```python
from build123d import *

# Parameters (mm, degrees)
BOSS_EXTRUDE1_DEPTH = 16.25
CUT_EXTRUDE1_DEPTH  = 1
SKETCH3_R           = 3.825
BOSS_EXTRUDE2_DEPTH = 3
CUT_EXTRUDE2_DEPTH  = 25.3
FILLET1_R           = 0.2
FILLET2_R           = 0.5
FILLET3_R           = 3
CUT_EXTRUDE3_DEPTH  = 4.45
CHAMFER1_SIZE       = 1.5


with BuildPart() as part:
    # Sketch1 → Boss-Extrude1 (new body, symmetric)
    with BuildSketch(Plane(origin=(0, 0, 0), x_dir=(0, 0, -1), z_dir=(1, 0, 0))):
        with BuildLine():
            Line((0, 0), (37.222256431, 0))
            ThreePointArc((37.222256431, 0), (44.515232504, 2.608290378), (48.5, 9.25))
            Line((48.5, 9.25), (44.35, 9.8))
            Line((44.35, 9.8), (44.35, 13.2))
            Line((44.35, 13.2), (48.5, 13.75))
            ThreePointArc((48.5, 13.75), (45.353984415, 19.631727984), (39.472256431, 22.777743569))
            Line((39.472256431, 22.777743569), (38.922256431, 18.627743569))
            Line((38.922256431, 18.627743569), (35.522256431, 18.627743569))
            Line((35.522256431, 18.627743569), (34.972256431, 22.777743569))
            ThreePointArc((34.972256431, 22.777743569), (30.886246606, 21.097133921), (27.735423451, 18))
            Line((27.735423451, 18), (0, 11.626817203))
            Line((0, 11.626817203), (0, 0))
        make_face()
    extrude(amount=BOSS_EXTRUDE1_DEPTH, both=True)

    # Sketch2 → Cut-Extrude1 (cut)
    with BuildSketch(Plane(origin=(16.25, 0, 0), x_dir=(0, 0, -1), z_dir=(1, 0, 0))):
        Polygon((24.85, 17.336973126), (24.85, 0), (48.5, 0), (48.5, 22.777743569), (24.85, 22.777743569), align=None)
    cut_extrude1 = extrude(amount=-CUT_EXTRUDE1_DEPTH, mode=Mode.SUBTRACT)

    # Sketch3 → Boss-Extrude2 (add)
    with BuildSketch(Plane(origin=(15.25, 0, 0), x_dir=(0, 0, -1), z_dir=(1, 0, 0))):
        with Locations((37.222256431, 11.5)):
            Circle(SKETCH3_R)
    boss_extrude2 = extrude(amount=BOSS_EXTRUDE2_DEPTH)

    # Mirror1: Cut-Extrude1, Boss-Extrude2 across plane
    add(cut_extrude1.mirror(Plane(origin=(0, 0, 0), x_dir=(0, 0, 1), z_dir=(1, 0, 0))), mode=Mode.SUBTRACT)
    add(boss_extrude2.mirror(Plane(origin=(0, 0, 0), x_dir=(0, 0, 1), z_dir=(1, 0, 0))))

    # Sketch4 → Cut-Extrude2 (cut)
    with BuildSketch(Plane(origin=(12.65, 0, 0), x_dir=(0, 0, -1), z_dir=(1, 0, 0))):
        Polygon((0, 1.1), (1.35, 1.1), (1.35, 2.7), (2.65, 2.7), (2.65, 0), (0, 0), align=None)
        Polygon((0, 3.45), (27, 3.45), (31.5, 0), (48.5, 0), (48.5, 22.777743569), (0, 22.777743569), align=None)
    extrude(amount=-CUT_EXTRUDE2_DEPTH, mode=Mode.SUBTRACT)

    # Fillet1
    fillet1_edges = [part.edges().sort_by_distance(p)[0] for p in [
        (-18.25, 11.5, -33.397256431),
        (18.25, 11.5, -33.397256431),
    ]]
    fillet(fillet1_edges, radius=FILLET1_R)

    # Fillet2
    fillet2_edges = [part.edges().sort_by_distance(p)[0] for p in [
        (-14.45, 0, 0),
        (-13.95, 22.777743569, -34.972256431),
        (-13.95, 22.777743569, -39.472256431),
        (-13.95, 13.75, -48.5),
        (-13.95, 9.25, -48.5),
        (14.45, 0, 0),
        (13.95, 22.777743569, -34.972256431),
        (13.95, 22.777743569, -39.472256431),
        (13.95, 13.75, -48.5),
        (13.95, 9.25, -48.5),
    ]]
    fillet(fillet2_edges, radius=FILLET2_R)

    # Fillet3
    fillet3_edges = [part.edges().sort_by_distance(p)[0] for p in [
        (-14.45, 11.626817203, 0),
        (14.45, 11.626817203, 0),
    ]]
    fillet(fillet3_edges, radius=FILLET3_R)

    # Sketch5 → Cut-Extrude3 (cut, through all)
    with BuildSketch(Plane(origin=(0, 3.45, 0), x_dir=(1, 0, 0), z_dir=(0, 1, 0))):
        with BuildLine():
            Line((-0.75, 4.75), (0.75, 4.75))
            ThreePointArc((0.75, 4.75), (3.5, 7.5), (0.75, 10.25))
            Line((0.75, 10.25), (-0.75, 10.25))
            ThreePointArc((-0.75, 10.25), (-3.5, 7.5), (-0.75, 4.75))
        make_face()
        with BuildLine():
            Line((7.75, 20.5), (6.25, 20.5))
            ThreePointArc((6.25, 20.5), (3.5, 17.75), (6.25, 15))
            Line((6.25, 15), (7.75, 15))
            ThreePointArc((7.75, 15), (10.5, 17.75), (7.75, 20.5))
        make_face()
        with BuildLine():
            Line((-7.75, 20.5), (-6.25, 20.5))
            ThreePointArc((-6.25, 20.5), (-3.5, 17.75), (-6.25, 15))
            Line((-6.25, 15), (-7.75, 15))
            ThreePointArc((-7.75, 15), (-10.5, 17.75), (-7.75, 20.5))
        make_face()
    extrude(amount=-CUT_EXTRUDE3_DEPTH, mode=Mode.SUBTRACT)

    # Chamfer1
    chamfer1_edges = [part.edges().sort_by_distance(p)[0] for p in [
        (-3.5, 3.45, -7.5),
        (0, 3.45, -4.75),
        (3.5, 3.45, -7.5),
        (0, 3.45, -10.25),
        (10.5, 3.45, -17.75),
        (7, 3.45, -20.5),
        (3.5, 3.45, -17.75),
        (7, 3.45, -15),
        (-10.5, 3.45, -17.75),
        (-7, 3.45, -15),
        (-3.5, 3.45, -17.75),
        (-7, 3.45, -20.5),
    ]]
    chamfer(chamfer1_edges, length=CHAMFER1_SIZE)


solid = part.part
```
Model file for the job. Use its own axes, mm. A direction names the side the tool comes from. Give positions to 0.01 mm unless a question says otherwise; leave off trailing zeros. Order: outer loops, then holes, each group sorted by start corner. A loop starts at its lowest first (then second) coordinate and runs counter-clockwise, first axis right, second up.
1) Saw through at A-A, the plane y = 6.5. Write the cut outline in (x, z).
2) Saw through at C-C, the plane z = -30.5. Write the cut outline in (x, y), then the cut area to 3 significant figures.
3) Saw through at B-B, the plane z = -7.5. Write the cut outline in (x, y).
4) Wall check: probe 1 along X at (y, z) = (16.75, -32.5); probe 2 along X at (y, z) = (10.75, -17); probe 3 along Z at (x, y) = (-8.5, 2.25). Give the ranges that are in metal, low to high.
5) Mould opens along Y. For faces 4 (the flat face through (-14, 11, -44.35)), 5 (the flat face through (16, 9, -24.85)), 6 (the cylindrical face through (-13.932, 2.368, -44.213)), 7 (the flat face through (-6.99, 2.69, -14.26)) say: +Y half, -Y half, draft (parallel to the pull), parting line (faces both ways), or undercut.
6) Saw through at D-D, the plane y = 11.5. Write the cut outline in (x, z), then the cut area to 3 significant figures.
7) 3-axis set-ups, long thin cutter, end or side, ignore diameter. For faces 1 (the conical face through (3.74, 2.19, -7.43)), 2 (the flat face through (0, 1, -10.25)), 3 (the flat face through (0, 2, -1.35)): which of +Z, -Z, +X, -X, +Y, -Y reach the whole face in a straight line?
8) Pin check, flat tips, straight feed: pin 1 (1.2 mm diameter, centred on x = 7, y = 1, fed in from -Z); pin 2 (6 mm diameter, centred on y = 11, z = -23.5, fed in from +X); pin 3 (2 mm diameter, centred on x = 0.5, z = -33, fed in from -Y); pin 4 (5 mm diameter, centred on y = 5.5, z = -13.5, fed in from -X). Stop position of each tip, or through.
Computed:
1. outline: (-16.25, -24.85) - (-15.25, -24.85) - (-15.25, -47.58) - (-12.65, -47.58) - (-12.65, 0) - (-16.25, 0) - close; (12.65, -47.58) - (15.25, -47.58) - (15.25, -24.85) - (16.25, -24.85) - (16.25, 0) - (12.65, 0) - close
2. outline: (-15.25, 0) - (15.25, 0) - (15.25, 20.83) - (12.65, 20.83) - (12.65, 0.77) - (-12.65, 0.77) - (-12.65, 20.83) - (-15.25, 20.83) - close
2. area: 128 mm2
3. outline: (-16.25, 0) - (-3.5, 0) - (-3.5, 1.95) - (-5, 3.45) - (-12.65, 3.45) - (-12.65, 13.35) - (-16.25, 13.35) - close; (3.5, 0) - (16.25, 0) - (16.25, 13.35) - (12.65, 13.35) - (12.65, 3.45) - (5, 3.45) - (3.5, 1.95) - close
4. probe 1: x = -15.25 to -12.65, 12.65 to 15.25
4. probe 2: x = -16.25 to -12.65, 12.65 to 16.25
4. probe 3: z = -28.57 to -20.71, -14.79 to -2.65, -1.35 to 0
5. face 4: undercut
5. face 5: draft
5. face 6: -Y half
5. face 7: +Y half
6. outline: (-18.25, -40.85) arc R0.2 ccw to (-18.05, -41.05) - (-15.25, -41.05) - (-15.25, -44.35) - (-12.65, -44.35) - (-12.65, -1.03) - (-16.25, -1.03) - (-16.25, -24.85) - (-15.25, -24.85) - (-15.25, -33.4) - (-18.05, -33.4) arc R0.2 ccw to (-18.25, -33.6) - close; (12.65, -44.35) - (15.25, -44.35) - (15.25, -41.05) - (18.05, -41.05) arc R0.2 ccw to (18.25, -40.85) - (18.25, -33.6) arc R0.2 ccw to (18.05, -33.4) - (15.25, -33.4) - (15.25, -24.85) - (16.25, -24.85) - (16.25, -1.03) - (12.65, -1.03) - close
6. area: 319 mm2
7. face 1: +Y
7. face 2: +Y, -Y
7. face 3: -Y
8. pin 1: stops at z = -30.98
8. pin 2: stops at x = 16.25
8. pin 3: passes through
8. pin 4: stops at x = -16.25
